```python
from build123d import *

# Parameters (mm, degrees)
SKETCH1_W        = 170
SKETCH1_H        = 359.85
EXTRUSION1_DEPTH = 6.35
HOLE2_D          = 4
HOLE2_DEPTH      = 8
HOLE2_TIP        = 1.201721238
HOLE3_D          = 5
HOLE3_DEPTH      = 8
HOLE3_TIP        = 1.502151548
HOLE4_D          = 9.75
HOLE4_DEPTH      = 5
HOLE5_D          = 11.2
HOLE5_DEPTH      = 6


with BuildPart() as part:
    # Sketch1 → Extrusion1 (new body)
    with BuildSketch(Plane(origin=(0, 0, 0), x_dir=(-1, 0, 0), z_dir=(0, 1, 0))):
        Rectangle(SKETCH1_W, SKETCH1_H)
    extrude(amount=EXTRUSION1_DEPTH)

    # Hole2
    with Locations(Plane(origin=(0, 0, 0), x_dir=(-1, 0, 0), z_dir=(0, -1, 0))):
        with Locations((19, -11), (-19, -11), (-19, 11), (19, 11)):
            Hole(HOLE2_D / 2, depth=HOLE2_DEPTH)
            with Locations((0, 0, -(HOLE2_DEPTH + HOLE2_TIP / 2))):  # 118° drill point
                Cone(0, HOLE2_D / 2, HOLE2_TIP, mode=Mode.SUBTRACT)

    # Hole3
    with Locations(Plane(origin=(0, 0, 0), x_dir=(-1, 0, 0), z_dir=(0, -1, 0))):
        with Locations((-42.5, -84.900000036), (-77.5, -84.900000036), (-42.5, -49.900000036), (-77.5, -49.900000036), (42.5, -49.900000036), (77.5, -49.900000036), (42.5, -84.900000036), (77.5, -84.900000036), (-77.5, 84.900000036), (-42.5, 84.900000036), (-77.5, 49.900000036), (-42.5, 49.900000036), (42.5, 84.900000036), (77.5, 84.900000036), (42.5, 49.900000036), (77.5, 49.900000036)):
            Hole(HOLE3_D / 2, depth=HOLE3_DEPTH)
            with Locations((0, 0, -(HOLE3_DEPTH + HOLE3_TIP / 2))):  # 118° drill point
                Cone(0, HOLE3_D / 2, HOLE3_TIP, mode=Mode.SUBTRACT)

    # Hole4
    with Locations(Plane(origin=(-19, 0, 11), x_dir=(0, 0, -1), z_dir=(0, -1, 0))):
        with Locations((0, 0), (0, 38), (22, 38), (22, 0)):
            Hole(HOLE4_D / 2, depth=HOLE4_DEPTH)

    # Hole5
    with Locations(Plane(origin=(-77.5, 0, 49.900000036), x_dir=(0, 0, -1), z_dir=(0, -1, 0))):
        with Locations((0, 0), (0, 35), (-35, 35), (-35, 0), (-35, 120), (-35, 155), (0, 155), (0, 120), (99.800000072, 155), (99.800000072, 120), (134.800000072, 120), (134.800000072, 155), (134.800000072, 35), (99.800000072, 35), (99.800000072, 0), (134.800000072, 0)):
            Hole(HOLE5_D / 2, depth=HOLE5_DEPTH)


solid = part.part
```
Could you check a few things on this model? Use its own coordinates, in mm. A direction names the side the tool comes from. Coordinates: 2 decimals unless noted, no trailing zeros. Answer as CSV lines item,"result". Start each with the question number.
1) For faces 1 (the flat face through (-85, 3, -3)), 2 (the flat face through (41.3, 6, 52.3)), which set-ups out of +Z, -Z, +X, -X, +Y, -Y let a thin tool reach every point of the face, with its end or its side?
2) I want a section at A-A, the plane y = 3.5. Give the number of separate pieces and of enclosed holes in the cut face, and give its area (3 significant figures).
3) We'd pull the mould along Z, two halves only. Please class faces 3 (the flat face through (18, 5, 13)), 4 (the flat face through (85, 3, -3)), 5 (the flat face through (1, 3, 179.925)): +Z half, -Z half, draft (parallel to the pull), parting line (faces both ways), or undercut.
4) For P1, Ø9, axis at x = -42.5, z = -49.9, coming from the -Y side; P2, Ø3, axis at x = 42.5, z = 49.9, coming from the -Y side; P3, Ø6.5, axis at x = 19, z = -11, coming from the -Y side, each with a flat end and sliding along its axis, tell me the tip position at first contact or that it passes through.
5) Please list where these lines run through material, in increasing order: line 1 (Z direction, x = -77.5, y = 6.3) (3 decimals); line 2 (Z direction, x = 19, y = 5.4) (3 decimals); line 3 (X direction, y = 5.7, z = 11). Write a range as from..to.
Data:
1,face 1,"+Z, -Z, -X, +Y, -Y"
1,face 2,"-Y"
2,separate pieces,"1"
2,enclosed holes,"20"
2,area,"59,300 mm^2"
3,face 3,"undercut"
3,face 4,"draft"
3,face 5,"+Z half"
4,P1,"stops at y = 6"
4,P2,"passes through"
4,P3,"stops at y = 5"
5,line 1,"z = -179.925..-87.4, -82.4..-52.4, -47.4..47.4, 52.4..82.4, 87.4..179.925"
5,line 2,"z = -179.925..-13, -9..9, 13..179.925"
5,line 3,"x = -85..-21, -17..17, 21..85"
